```python
from build123d import *

# Parameters (mm, degrees)
F1_DEPTH = 17
F3_DEPTH = 7.75
F5_DEPTH = 5
F7_DEPTH = 25


with BuildPart() as f1:
    # F0 (on Top) → F1 (new body)
    with BuildSketch(Plane.XY):
        Polygon((0, -64.15), (0, 0), (-63.45, 0), (-63.45, 7.65), (-53.45, 7.65), (-53.45, 12.65), (-68.45, 12.65), (-68.45, -5), (-5, -5), (-5, -69.15), (12.75, -69.15), (12.75, -54.15), (7.75, -54.15), (7.75, -64.15), align=None)
    extrude(amount=F1_DEPTH)

    # F2 (on face) → F3 (join)
    with BuildSketch(Plane.YZ):
        Polygon((-58.58, 17), (-64.15, 17), (-64.15, 0), align=None)
    extrude(amount=F3_DEPTH)

    # F4 (on face) → F5 (join)
    with BuildSketch(Plane.YZ.offset(12.75)):
        Polygon((-48.58, 17), (-54.15, 17), (-54.15, 0), align=None)
    extrude(amount=-F5_DEPTH)

    # F6 (on face) → F7 (cut)
    with BuildSketch(Plane.YZ.offset(12.75)):
        Polygon((-63.58, 17), (-69.15, 17), (-69.15, 0), align=None)
    extrude(amount=-F7_DEPTH, mode=Mode.SUBTRACT)


solid = f1.part
```
For this review, take the finished solid that the model builds, in its own axes (mm). A direction names the side the tool comes from. Give positions to 0.01 mm unless a question says otherwise; leave off trailing zeros. Write each loop counter-clockwise with the first axis right and the second up, starting at its lowest first coordinate (ties: lowest second). Pieces come first, ordered by that corner, then holes. Notation, with made-up numbers: M 71,70 L 125,70 A18 cw 125,104 Z; hole C 64.25,47.5 d3. An arc over 180 degrees is marked long. Answer as CSV lines item,"result".
1. Consider section A-A, the plane x = -56. Write out the cut boundary in (y, z), then the cut area to 3 significant figures.
Findings:
outline,"M -5,0 L 0,0 L 0,17 L -5,17 Z; M 7.65,0 L 12.65,0 L 12.65,17 L 7.65,17 Z"
area,"170 mm2"
2. For faces 5 (the flat face through (-53.45, 10, 8)), 6 (the flat face through (10.285, -51.404, 8.381)), 7 (the flat face through (7.75, -56, 9)), 8 (the flat face through (-5, -37, 8)), list the 3-axis set-ups (+Z, -Z, +X, -X, +Y, -Y) from which the entire face can be reached by the end or side of a thin tool; tool diameter is ignored.
Findings:
face 5,"+Z, -Z, +X, +Y"
face 6,"-Z, +X, +Y"
face 7,"-Z, +Y"
face 8,"+Z, -Z, -X, -Y"
3. Draft analysis for pull direction Y (two halves, no side actions). For faces 1 (the flat face through (-59, 7.65, 8)), 2 (the flat face through (12.75, -59, 9)), 3 (the flat face through (-63.45, 4, 8)), 4 (the flat face through (-37, -5, 8)), state which applies: +Y half, -Y half, draft (parallel to the pull), parting line (faces both ways), or undercut.
Findings:
face 1,"undercut"
face 2,"draft"
face 3,"undercut"
face 4,"-Y half"
4. Consider section B-B, the plane z = 3.25. Write out the cut boundary in (x, y).
Findings:
outline,"M -68.45,-5 L -5,-5 L -5,-68.09 L 12.75,-68.09 L 12.75,-53.09 L 7.75,-53.09 L 7.75,-63.09 L 0,-63.09 L 0,0 L -63.45,0 L -63.45,7.65 L -53.45,7.65 L -53.45,12.65 L -68.45,12.65 Z"
5. For pin 1 (4 mm diameter, centred on x = -43, z = 10.5, fed in from -Y); pin 2 (3 mm diameter, centred on x = -15.5, z = 14, fed in from +Y); pin 3 (4 mm diameter, centred on y = 2.5, z = 7, fed in from +X), all flat-tipped, find the tip position at first contact; note any pin that passes through.
Findings:
pin 1,"stops at y = -5"
pin 2,"stops at y = 0"
pin 3,"stops at x = -63.45"
6. Consider section C-C, the plane y = -2. Write out the cut boundary in (x, z), then the cut area to 3 significant figures.
Findings:
outline,"M -68.45,0 L 0,0 L 0,17 L -68.45,17 Z"
area,"1,160 mm2"
7. Wall thickness on line 1 (Y direction, x = -55, z = 12); line 2 (Y direction, x = -32, z = 10.5): over which ranges is each line inside the solid? List them lowest first.
Findings:
line 1,"y = -5 to 0, 7.65 to 12.65"
line 2,"y = -5 to 0"
8. Consider section D-D, the plane x = -39. Write out the cut boundary in (y, z).
Findings:
outline,"M -5,0 L 0,0 L 0,17 L -5,17 Z"
